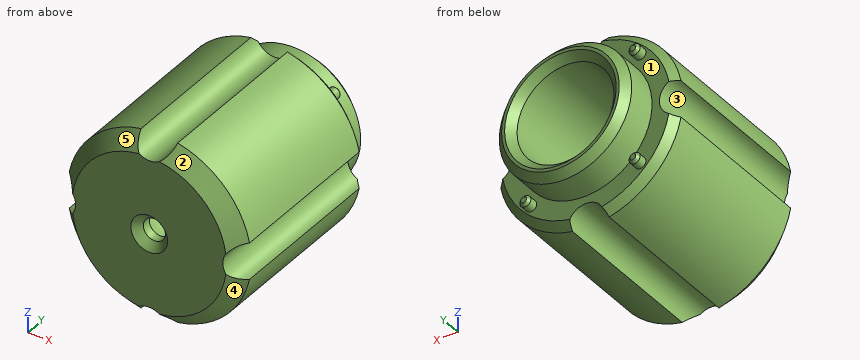
Autodesk Inventor part; units mm, degrees
ref_plane "YZ Plane" through (0, 0, 0) normal (1, 0, 0) x (0, 1, 0)
ref_plane "XZ Plane" through (0, 0, 0) normal (0, 1, 0) x (-1, 0, 0)
ref_plane "XY Plane" through (0, 0, 0) normal (0, 0, 1) x (1, 0, 0)
sketch "Sketch1" plane through (0, 0, 0) normal (0, 0, 1) x (1, 0, 0)
  line L0 (0, 0) -> (42.0469, 0) construction
  line L1 (0, 0) -> (0, 27.7015) construction
  arc A0 (0, -6.6) -> (6.5875, 0.406) centre (0, 0) ccw
  line L2 (6.5875, 0.406) -> (6.5875, 16)
  line L3 (6.5875, 16) -> (9, 16)
  line L4 (9, 16) -> (9, 21)
  line L5 (9, 21) -> (12.5, 21)
  line L6 (12.5, 21) -> (12.5, -8.6)
  line L7 (12.5, -8.6) -> (0, -8.6)
  line L8 (0, -8.6) -> (0, -6.6)
  line L9 (9, 16) -> (6.5875, 16)
  line L10 (6.5875, 16) -> (6.5875, 21)
  line L11 (6.5875, 21) -> (9, 21)
  line L12 (9, 21) -> (9, 16)
  line L13 (12.5, 16) -> (9, 16)
  line L14 (2, -8.6) -> (0, -8.6)
  line L15 (0, -8.6) -> (0, -6.6)
  dimension "d0" = 13.2
  dimension "d2" = 5
  dimension "d3" = 9
  dimension "d4" = 12.5
  dimension "d5" = 6.5875
  dimension "d6" = 2
  dimension "d35" = 16
revolve "Revolution1" add sketch "Sketch1" angle 360 about axis through (0, 0, 0) along (0, 1, 0) contours A0 L2 L3 L13 L6 L7 L8 | L10 L11 L4 L3
chamfer "Chamfer1" distance 2 angle 45 1 edges at (-12.5, -8.6, 0)
chamfer "Chamfer3" distance 1 angle 45 3 edges at (-9, 21, 0) (-12.5, 16, 0) (-6.5875, 21, 0)
sketch "Sketch2" plane through (0, 16, 0) normal (0, 1, 0) x (1, 0, 0)
  circle A0 centre (0, 0) radius 10.5 construction
  line L0 (0, 0) -> (0, 17.3905) construction
  line L1 (0, 0) -> (14.2747, 14.2747) construction
  circle A1 centre (7.4246, 7.4246) radius 0.75
  circle A2 centre (0, 0) radius 12.5
  circle A3 centre (0, 0) radius 12.5
  circle A4 centre (0, 12.5) radius 2.5
  point P0 (-2.4875, 12.25)
  point P1 (2.4875, 12.25)
  dimension "d17" = 21
  dimension "d29" = 25
  dimension "d18" = 45
  dimension "d19" = 1.5
  dimension "d28" = 5
extrude "Extrusion1" add sketch "Sketch2" along normal blind 1.5 contours A1
chamfer "Chamfer4" distance 0.35 angle 45 1 edges at (6.6746, 17.5, -7.4246)
extrude "Extrusion2" cut sketch "Sketch2" against normal through all contours A4 A2 picked at (0, 11.6481)
pattern_circular "Circular Pattern2" count 4 over 360 about axis through (0, -10, 0) along (0, 1, 0) of "Extrusion1", "Extrusion2", "Chamfer4"
sketch "Sketch3" plane through (0, -8.6, -12.5) normal (0, -1, 0) x (1, 0, 0)
  circle A0 centre (0, 12.5) radius 1.5
  dimension "d37" = 3
extrude "Extrusion3" cut sketch "Sketch3" against normal through all
chamfer "Chamfer5" distance 1 angle 45 1 edges at (-1.5, -8.6, 0)
properties part number "centrifugetool_5mm_tubecap_v2"
Could you check a few things on this model? Use its own coordinates, in mm. Face numbers are marked on the shaded views. A direction names the side the tool comes from. Give positions to 0.01 mm unless a question says otherwise; leave off trailing zeros. Put each result on its own line as item: value.
(1) Thinking about a two-plate mould opening in Z: for the marked faces 3, 4 and 5, which applies, pulls with the +Z half, pulls with the -Z half, needs draft (parallel to the pull), parting line crosses it, or undercut?
Computed:
face 3: undercut
face 4: pulls with the -Z half
face 5: pulls with the +Z half
(2) I'm going to push flat-ended pins straight in: pin 1 Ø0.6 at (x, z) = (7.5, 7.5) entering from +Y; pin 2 Ø6 at (x, y) = (8, 13) entering from -Z; pin 3 Ø1 at (x, y) = (-0.5, 15) entering from +Z. Where does each tip first touch, or does it pass through?
Computed:
pin 1: y = 17.5
pin 2: z = -11.46
pin 3: z = 10.21
(3) Please list where these lines run through material, in increasing order: probe 1 along Z at (x, y) = (0, -7.3); probe 2 along Z at (x, y) = (0, 13.25). Write a range as [from, to].
Computed:
probe 1: [-10, -1.5], [1.5, 10]
probe 2: [-10, -6.59], [6.59, 10]
(4) For the marked faces 1 and 2, which set-ups out of +Z, -Z, +X, -X, +Y, -Y let a thin tool reach every point of the face, with its end or its side?
Computed:
face 1: +Y
face 2: +Z, +X, -Y
